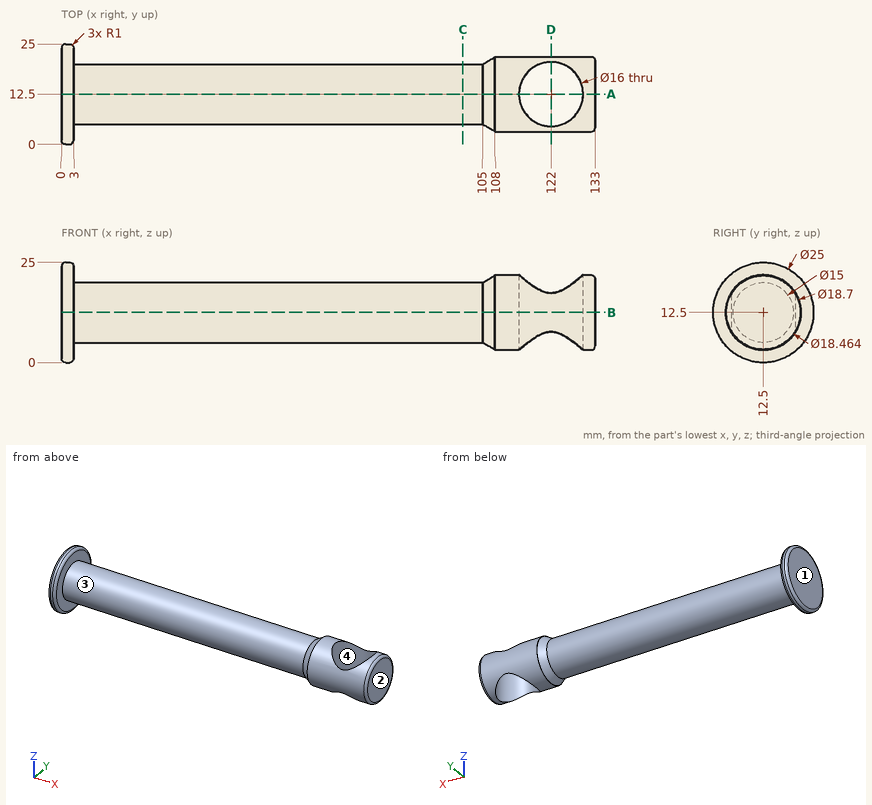
Geometry: see drawing. Coordinates: mm, zero at the bounding-box minimum. Coordinates: 2 decimals unless noted, no trailing zeros. Order: outer loops, then holes, each group sorted by start corner. A loop starts at its lowest first (then second) coordinate and runs counter-clockwise, first axis right, second up. Notation, with made-up numbers: (4, -27) - (54, -27) arc R14 ccw to (54, -18) - close; hole circle Ø10 at (58.25, -39). An arc over 180 degrees is marked (long way). Return JSON: item names as keys, results as strings.
Q1. Cut plane D-D (x = 122). Return loops of the section in (y, z), then the cut area to 3 significant figures.
The answers:
{"outline": "(4.5, 7.66) - (4.5, 17.34) arc R9.35 ccw to start; (20.5, 7.66) arc R9.35 ccw to (20.5, 17.34) - close", "area": "17.7 mm2"}
Q2. Cut plane B-B (z = 12.5). Return loops of the section in (x, y).
The answers:
{"outline": "(0, 1) arc R1 ccw to (1, 0) - (2, 0) arc R1 ccw to (3, 1) - (3, 5) - (105, 5) - (108, 3.27) - (108, 3.15) - (132, 3.15) arc R1 ccw to (133, 4.15) - (133, 20.85) arc R1 ccw to (132, 21.85) - (108, 21.85) - (108, 21.73) - (105, 20) - (3, 20) - (3, 24) arc R1 ccw to (2, 25) - (1, 25) arc R1 ccw to (0, 24) - close; hole circle Ø16 at (122, 12.5)"}
Q3. First-contact query: pin 1 (12 mm diameter, centred on x = 46, y = 13, fed in from +Z); pin 2 (12 mm diameter, centred on x = 54, z = 18.5, fed in from +Y). Flat tips, straight axial feed; report the tip coordinate or a pass-through.
The answers:
{"pin 1": "stops at z = 20", "pin 2": "stops at y = 20"}
Q4. Draft query along X for the marked faces 1, 2, 3 and 4. Return one class per face: +X half, -X half, draft (parallel to the pull), parting line (faces both ways), or undercut.
The answers:
{"face 1": "-X half", "face 2": "+X half", "face 3": "undercut", "face 4": "undercut"}
Q5. Ray query, probe 1 along Y at (x, z) = (122, 12.5); probe 2 along X at (y, z) = (12.5, 13.25); probe 3 along Y at (x, z) = (122, 8.25). Return the intervals inside material, ascending.
The answers:
{"probe 1": "y = 3.15 to 4.5, 20.5 to 21.85", "probe 2": "x = 0 to 114, 130 to 133", "probe 3": "y = 4.17 to 4.5, 20.5 to 20.83"}
Q6. Cut plane C-C (x = 100). Return loops of the section in (y, z), then the cut area to 3 significant figures.
The answers:
{"outline": "circle Ø15 at (12.5, 12.5)", "area": "177 mm2"}
Q7. Cut plane A-A (y = 12.5). Return loops of the section in (x, z), then the cut area to 3 significant figures.
The answers:
{"outline": "(0, 1) arc R1 ccw to (1, 0) - (2, 0) arc R1 ccw to (3, 1) - (3, 5) - (105, 5) - (108, 3.27) - (108, 3.15) - (114, 3.15) - (114, 21.85) - (108, 21.85) - (108, 21.73) - (105, 20) - (3, 20) - (3, 24) arc R1 ccw to (2, 25) - (1, 25) arc R1 ccw to (0, 24) - close; (130, 3.15) - (132, 3.15) arc R1 ccw to (133, 4.15) - (133, 20.85) arc R1 ccw to (132, 21.85) - (130, 21.85) - close", "area": "1,820 mm2"}
